Input: part model. Units: mm. Frame: model coordinates. A direction names the side the tool comes from. Round coordinates to 2 decimals unless told otherwise and drop trailing zeros. Loops run counter-clockwise (first coordinate to the right, second up) from the corner with the lowest first, then second, coordinate; pieces in that order, holes last. Notation, with made-up numbers: M 50.25,33.25 L 94.25,33.25 A24 cw 94.25,61.25 Z; hole C 53,-4.75 d8. An arc over 180 degrees is marked long. Use one line per item in the form item = value. Start each with the question number.
Q1. Ray query, line 1 along X through (y, z) = (0.5, -52); line 2 along Z through (x, y) = (-1.5, 6.75); line 3 along Y through (x, z) = (0, -27). Return the intervals inside material, ascending.
Q2. Access query for faces 5 (the flat face through (3.969, 0, 55)), 6 (the flat face through (8, -3, 49.212)), 7 (the cylindrical face through (-8.2, -7.5, 53.5)). Directions: +Z, -Z, +X, -X, +Y, -Y. A direction counts if a zero-diameter tool reaches every point of the face in a straight line with its end or side. Return the directions, or none.
Q3. First-contact query: P1, Ø3, axis at x = -5.5, z = 32, coming from the -Y side; P2, Ø2, axis at x = 5, z = 1, coming from the +Y side; P3, Ø12, axis at x = 8, y = -3, coming from the -Z side; P4, Ø1, axis at x = -8.5, y = -7, coming from the -Z side. Flat tips, straight axial feed; report the tip coordinate or a pass-through.
Q4. Section query A-A, the plane z = 1.5. Output: boundary loops of the cut face in (x, y) (1 decimal).
Q5. Mould query, pull axis Z, two halves, no side actions, for faces 1 (the cylindrical face through (-7.533, -0.332, 48.042)), 2 (the cylindrical face through (0.66, -5, -42.32)), 3 (the conical face through (2.163, -3.683, 58.426)), 4 (the cylindrical face through (-1.72, 7.75, 4.45)). Classes: pulls with the +Z half, pulls with the -Z half, needs draft (parallel to the pull), parting line crosses it, or undercut.
```python
from build123d import *

# Parameters (mm, degrees)
CUT_EXTRUDE1_DEPTH = 7.14375


with BuildPart() as part:
    # Sketch4 → Revolve1 (revolve)
    with BuildSketch(Plane(origin=(0, 0, 0), x_dir=(0, 0, -1), z_dir=(1, 0, 0)), mode=Mode.PRIVATE) as revolve1_sk:
        Polygon((-49.2125, 11.1125), (-57.62625, 11.1125), (-58.7375, 10.00125), (-58.7375, 0), (39.6875, 0), (39.6875, 7.408333333), (39.158333333, 7.9375), (-46.8503, 7.9375), (-47.247175, 7.540625), (-48.815625, 7.540625), (-49.2125, 7.9375), align=None)
    revolve(revolve1_sk.sketch.rotate(Axis((0, 0, 58.7375), (0, 0, -1)), 90), axis=Axis((0, 0, 58.7375), (0, 0, -1)))

    # Sketch5 → Cut-Extrude1 (cut)
    with BuildSketch(Plane.XY.offset(58.7375)):
        Polygon((3.96875, 2.291358881), (0, 4.582717762), (-3.96875, 2.291358881), (-3.96875, -2.291358881), (0, -4.582717762), (3.96875, -2.291358881), align=None)
    extrude(amount=-CUT_EXTRUDE1_DEPTH, mode=Mode.SUBTRACT)

    # Cut-Extrude4 cone 1 section (on through the dimple's axis) → Cut-Extrude4 (revolve, cut)
    with BuildSketch(Plane(origin=(0, 0, 58.7375), x_dir=(0, -1, 0), z_dir=(1, 0, 0))):
        Polygon((0, 0), (4.582717762, 0), (0, 4.582717762), align=None)
    revolve(axis=Axis((0, 0, 58.7375), (0, 0, -1)), mode=Mode.SUBTRACT)

    # Sketch7 → Revolve2 (revolve)
    with BuildSketch(Plane(origin=(0, 0, 0), x_dir=(0, 0, -1), z_dir=(1, 0, 0)), mode=Mode.PRIVATE) as revolve2_sk:
        Polygon((39.6875, 6.35), (57.272115385, 6.35), (58.7375, 4.884615385), (58.7375, 0), (39.6875, 0), align=None)
    revolve(revolve2_sk.sketch.rotate(Axis((0, 0, -58.7375), (0, 0, 1)), 90), axis=Axis((0, 0, -58.7375), (0, 0, 1)))

    # Sketch10 → Cut-Revolve1 (revolve, cut)
    with BuildSketch(Plane(origin=(0, 0, 0), x_dir=(0, 0, -1), z_dir=(1, 0, 0)), mode=Mode.PRIVATE) as cut_revolve1_sk:
        with BuildLine():
            Line((40.9956, 5.0419), (43.5991, 5.0419))
            Line((43.5991, 5.0419), (46.4947, 7.9375))
            Line((46.4947, 7.9375), (39.6875, 7.9375))
            Line((39.6875, 7.9375), (39.6875, 6.35))
            ThreePointArc((39.6875, 6.35), (40.07063362, 5.42503362), (40.9956, 5.0419))
        make_face()
    revolve(cut_revolve1_sk.sketch.rotate(Axis((0, 0, -58.7375), (0, 0, 1)), 90), axis=Axis((0, 0, -58.7375), (0, 0, 1)), mode=Mode.SUBTRACT)


solid = part.part
```
Results found:
q1.line_1 = -6.33 to 6.33
q1.line_2 = -39.69 to 58.74
q1.line_3 = -7.94 to 7.94
q2.face_5 = +Z
q2.face_6 = -Z
q2.face_7 = +Z, -Z
q3.P1 = -6.86
q3.P2 = 6.86
q3.P3 = -58.74
q3.P4 = 49.21
q4.outline = C 0,0 d15.9
q5.face_1 = undercut
q5.face_2 = undercut
q5.face_3 = pulls with the +Z half
q5.face_4 = needs draft
